Here's the drawing with two shaded views (mm, measured from the low corner). I have some questions. A direction names the side the tool comes from. Give positions to 0.01 mm unless a question says otherwise; leave off trailing zeros. Write each loop counter-clockwise with the first axis right and the second up, starting at its lowest first coordinate (ties: lowest second). Pieces come first, ordered by that corner, then holes. Notation, with made-up numbers: (73, 25) - (106, 25) arc R33 ccw to (106, 56) - close; hole circle Ø6 at (56.25, 39.5). An arc over 180 degrees is marked (long way). Use one line per item in the form item = value.
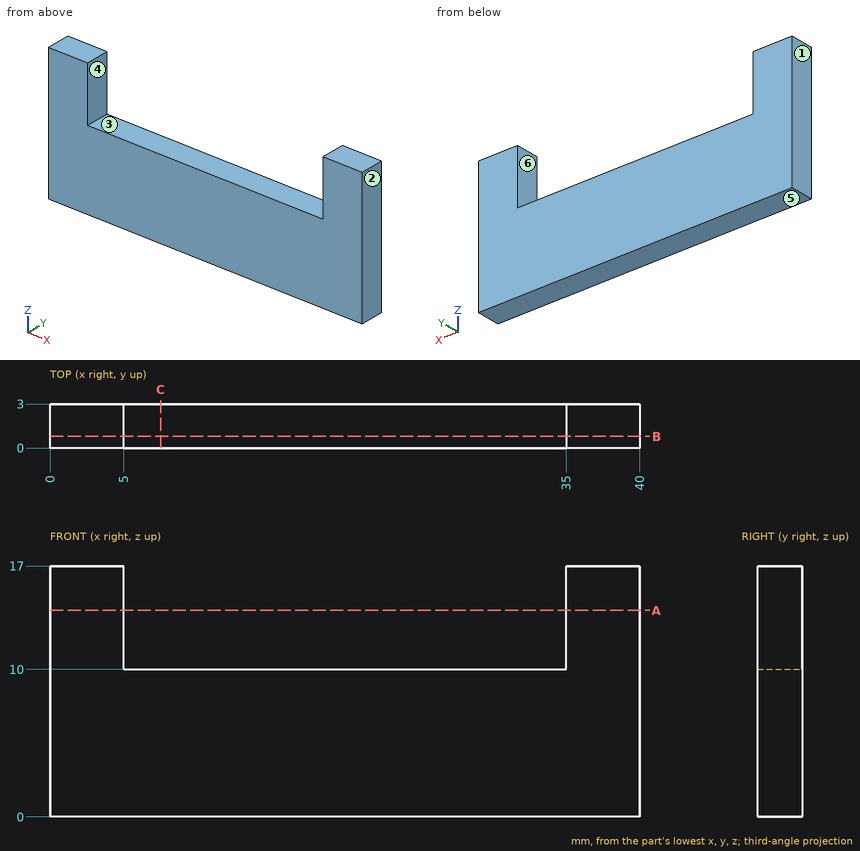
1. Which directions (+Z, -Z, +X, -X, +Y, -Y) give clear straight access to the entire face, cutting with the end or side of a thin tool? Please do the marked faces 5 and 6.
Response values:
face_5 = -Z, +X, -X, +Y, -Y
face_6 = +Z, +Y, -Y
2. Imagine slicing it at C-C, the plane x = 7.5. List the corners of the cut face in (y, z) for me, and give its area (3 significant figures).
Response values:
outline = (0, 0) - (3, 0) - (3, 10) - (0, 10) - close
area = 30.0 mm²
3. If we mould it in two halves opening along X, with no side actions, what happens to the marked faces 1, 2, 3 and 4? For each: pulls with the +X half, pulls with the -X half, needs draft (parallel to the pull), parting line crosses it, or undercut.
Response values:
face_1 = pulls with the -X half
face_2 = pulls with the +X half
face_3 = undercut
face_4 = undercut
4. For pin 1 (1 mm diameter, centred on y = 2.5, z = 6, fed in from -X); pin 2 (1.5 mm diameter, centred on x = 22, y = 1, fed in from +Z), each with a flat end and sliding along its axis, tell me the tip position at first contact or that it passes through.
Response values:
pin_1 = 0
pin_2 = 10
5. If I drill on line 1 (Z direction, x = 15, y = 2.1); line 2 (X direction, y = 0.6, z = 12.5), over which ranges is the centre line in solid material (lowest first)? Write a range as from..to.
Response values:
line_1 = 0..10
line_2 = 0..5, 35..40
6. Imagine slicing it at B-B, the plane y = 0.8. List the corners of the cut face in (x, z) for me.
Response values:
outline = (0, 0) - (40, 0) - (40, 17) - (35, 17) - (35, 10) - (5, 10) - (5, 17) - (0, 17) - close
7. Imagine slicing it at A-A, the plane z = 14. List the corners of the cut face in (x, y) for me, and give its area (3 significant figures).
Response values:
outline = (0, 0) - (5, 0) - (5, 3) - (0, 3) - close; (35, 0) - (40, 0) - (40, 3) - (35, 3) - close
area = 30.0 mm²
